```python
from build123d import *

# Parameters (mm, degrees)
F0_W     = 279.4
F0_H     = 482.6
F1_DEPTH = 25.4
F2_W     = 177.8
F2_H     = 17.78
F3_DEPTH = 25.4
F4_W     = 25.4
F4_H     = 25.4
F5_DEPTH = 17.78
F4_W_2   = 127
F4_H_2   = 127
F6_DEPTH = 12.7


with BuildPart() as f1:
    # F0 (on Front) → F1 (new body)
    with BuildSketch(Plane.XZ):
        with Locations((-3.365506, 53.583339)):
            Rectangle(F0_W, F0_H)
    extrude(amount=F1_DEPTH)

    # F2 (on face) → F3 (cut)
    with BuildSketch(Plane.XZ.offset(25.4)):
        with Locations((-3.365506, 235.193339)):
            Rectangle(F2_W, F2_H)
        with Locations((-3.365506, 192.013339)):
            Rectangle(F2_W, F2_H)
    extrude(amount=-F3_DEPTH, mode=Mode.SUBTRACT)

    # F4 (on face) → F5 (join)
    with BuildSketch(Plane.XZ.offset(25.4)):
        with Locations((34.734494, -101.6)):
            Rectangle(F4_W, F4_H)
        with Locations((72.834494, -101.6)):
            Rectangle(F4_W, F4_H)
        with Locations((110.934494, -101.6)):
            Rectangle(F4_W, F4_H)
        with Locations((110.934494, -63.5)):
            Rectangle(F4_W, F4_H)
        with Locations((72.834494, -63.5)):
            Rectangle(F4_W, F4_H)
        with Locations((34.734494, -63.5)):
            Rectangle(F4_W, F4_H)
        with Locations((34.734494, -25.4)):
            Rectangle(F4_W, F4_H)
        with Locations((72.834494, -25.4)):
            Rectangle(F4_W, F4_H)
        with Locations((110.934494, -25.4)):
            Rectangle(F4_W, F4_H)
    extrude(amount=F5_DEPTH)

    # F4 (on face) → F6 (join)
    with BuildSketch(Plane.XZ.offset(25.4)):
        with Locations((72.834494, -63.5)):
            Rectangle(F4_W_2, F4_H_2)
        with Locations((34.734494, -101.6)):
            Rectangle(F4_W, F4_H, mode=Mode.SUBTRACT)
        with Locations((72.834494, -101.6)):
            Rectangle(F4_W, F4_H, mode=Mode.SUBTRACT)
        with Locations((110.934494, -101.6)):
            Rectangle(F4_W, F4_H, mode=Mode.SUBTRACT)
        with Locations((34.734494, -63.5)):
            Rectangle(F4_W, F4_H, mode=Mode.SUBTRACT)
        with Locations((34.734494, -25.4)):
            Rectangle(F4_W, F4_H, mode=Mode.SUBTRACT)
        with Locations((72.834494, -63.5)):
            Rectangle(F4_W, F4_H, mode=Mode.SUBTRACT)
        with Locations((72.834494, -25.4)):
            Rectangle(F4_W, F4_H, mode=Mode.SUBTRACT)
        with Locations((110.934494, -63.5)):
            Rectangle(F4_W, F4_H, mode=Mode.SUBTRACT)
        with Locations((110.934494, -25.4)):
            Rectangle(F4_W, F4_H, mode=Mode.SUBTRACT)
    extrude(amount=F6_DEPTH)


solid = f1.part
```
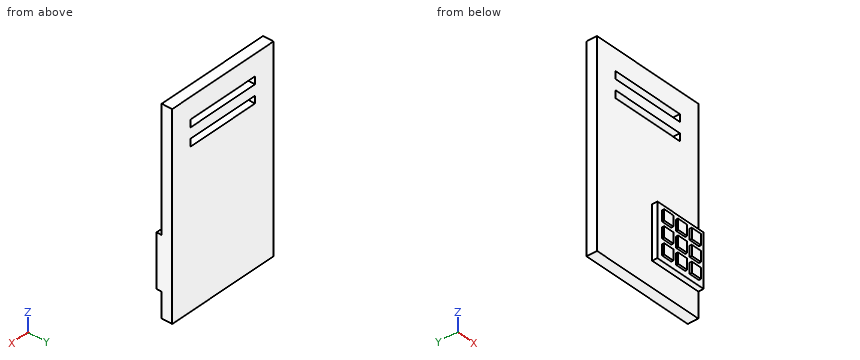
Work out the finished part from the listing and answer in its coordinate system (mm). Give positions to 0.01 mm unless a question says otherwise; leave off trailing zeros. Loops run counter-clockwise (first coordinate to the right, second up) from the corner with the lowest first, then second, coordinate; pieces in that order, holes last. Notation, with made-up numbers: (82, 66.5) -> (123, 66.5) arc R16 cw to (123, 93.5) -> close; hole circle Ø2 at (83.25, 4). An arc over 180 degrees is marked (long way). Write item = value, one per line. Start each with the question number.
(1) Find section C-C on x = 67. Give the vertices of the cut face in (y, z).
(2) Find section A-A on x = 16. Give the vertices of the cut face in (y, z), and give its area (3 significant figures).
(3) Find section B-B on y = -12. Give the vertices of the cut face in (x, z).
(4) Given pin 1 Ø10 at (x, y) = (-45.5, -30) entering from +Z; pin 2 Ø1.5 at (y, z) = (-41.5, -21) entering from -X; pin 3 Ø5.5 at (y, z) = (-41, -28) entering from +X; pin 4 Ø2.5 at (x, y) = (70, -41) entering from -Z, each flat-ended and moving along its own axis, determine where each tip first touches the part or whether it passes through.
(5) Find section D-D on z = 258. Give the vertices of the cut face in (x, y), and give its area (3 significant figures).
(6) Find the intervals of material crossed by probe 1 along Z at (x, y) = (31, -10.5); probe 2 along Z at (x, y) = (95.5, -35); probe 3 along X at (y, z) = (-37, -30.5), in increasing order. Write a range as from..to.
From the geometry:
q1.outline = (-43.18, -114.3) -> (-38.1, -114.3) -> (-38.1, -127) -> (-25.4, -127) -> (-25.4, -187.72) -> (0, -187.72) -> (0, 183.12) -> (-25.4, 183.12) -> (-25.4, 0) -> (-38.1, 0) -> (-38.1, -12.7) -> (-43.18, -12.7) -> (-43.18, -38.1) -> (-38.1, -38.1) -> (-38.1, -50.8) -> (-43.18, -50.8) -> (-43.18, -76.2) -> (-38.1, -76.2) -> (-38.1, -88.9) -> (-43.18, -88.9) -> close; (-25.4, 200.9) -> (0, 200.9) -> (0, 226.3) -> (-25.4, 226.3) -> close; (-25.4, 244.08) -> (0, 244.08) -> (0, 294.88) -> (-25.4, 294.88) -> close
q2.outline = (-38.1, -127) -> (-25.4, -127) -> (-25.4, -187.72) -> (0, -187.72) -> (0, 183.12) -> (-25.4, 183.12) -> (-25.4, 0) -> (-38.1, 0) -> close; (-25.4, 200.9) -> (0, 200.9) -> (0, 226.3) -> (-25.4, 226.3) -> close; (-25.4, 244.08) -> (0, 244.08) -> (0, 294.88) -> (-25.4, 294.88) -> close
q2.area = 13,000 mm^2
q3.outline = (-143.07, -187.72) -> (136.33, -187.72) -> (136.33, 294.88) -> (-143.07, 294.88) -> close; hole (-92.27, 183.12) -> (85.53, 183.12) -> (85.53, 200.9) -> (-92.27, 200.9) -> close; hole (-92.27, 226.3) -> (85.53, 226.3) -> (85.53, 244.08) -> (-92.27, 244.08) -> close
q4.pin_1 = 294.88
q4.pin_2 = 22.03
q4.pin_3 = 123.63
q4.pin_4 = -114.3
q5.outline = (-143.07, -25.4) -> (136.33, -25.4) -> (136.33, 0) -> (-143.07, 0) -> close
q5.area = 7,100 mm^2
q6.probe_1 = -187.72..183.12, 200.9..226.3, 244.08..294.88
q6.probe_2 = -127..0
q6.probe_3 = 9.33..136.33
